Input: part model. Units: mm. Frame: model coordinates. Coordinates: 2 decimals unless noted, no trailing zeros. Loops run counter-clockwise (first coordinate to the right, second up) from the corner with the lowest first, then second, coordinate; pieces in that order, holes last. Notation, with made-up numbers: (47, 70.25) - (100, 70.25) arc R16 ccw to (100, 86.25) - close; hole circle Ø2 at (-33, 50.5). An arc over 180 degrees is marked (long way). Write item = value, one per line. Start each with the question number.
Autodesk Inventor part; units mm, degrees
ref_plane "YZ Plane" through (0, 0, 0) normal (1, 0, 0) x (0, 1, 0)
ref_plane "XZ Plane" through (0, 0, 0) normal (0, 1, 0) x (-1, 0, 0)
ref_plane "XY Plane" through (0, 0, 0) normal (0, 0, 1) x (1, 0, 0)
sketch "Sketch1" plane through (0, 0, 0) normal (0, 0, 1) x (1, 0, 0)
  line L0 (3.175, 0) -> (3.175, 3.175)
  line L1 (3.175, 3.175) -> (-3.175, 3.175)
  line L2 (-3.175, 3.175) -> (-3.175, 0)
  line L3 (5.08, 0) -> (5.08, 5.08)
  line L4 (5.08, 5.08) -> (-5.08, 5.08)
  line L5 (-5.08, 5.08) -> (-5.08, 0)
  line L6 (-5.08, 0) -> (-3.175, 0)
  line L7 (3.175, 0) -> (5.08, 0)
  point P0 (0, 0)
  dimension "d0" = 6.35
  dimension "d1" = 3.175
  dimension "d2" = 10.16
  dimension "d3" = 5.08
extrude "Extrusion1" add sketch "Sketch1" along normal blind 215.9
sketch "Sketch2" plane through (-5.08, 5.08, 0) normal (0, 1, 0) x (1, 0, 0)
  circle A0 centre (5.08, -6.35) radius 1.985
  circle A1 centre (5.08, -209.55) radius 1.985
  circle A2 centre (5.08, -44.45) radius 1.985
  circle A3 centre (5.08, -171.45) radius 1.985
  circle A4 centre (5.08, -95.25) radius 1.985
  circle A5 centre (5.08, -120.65) radius 1.985
  point P0 (5.08, 0)
  dimension "d6" = 3.97
  dimension "d7" = 3.97
  dimension "d8" = 3.97
  dimension "d9" = 3.97
  dimension "d10" = 3.97
  dimension "d11" = 3.97
extrude "Extrusion2" cut sketch "Sketch2" against normal blind 215.9
sketch "Sketch3" plane through (5.08, 0, 0) normal (1, 0, 0) x (0, 0, -1)
  point P0 (0, 0)
sketch "Sketch4" plane through (-5.08, 5.08, 0) normal (0, 1, 0) x (1, 0, 0)
  circle A0 centre (5.08, -6.35) radius 1.985
  circle A1 centre (5.08, -44.45) radius 1.985
  circle A2 centre (5.08, -95.25) radius 1.985
  circle A3 centre (5.08, -120.65) radius 1.985
  circle A4 centre (5.08, -171.45) radius 1.985
  circle A5 centre (5.08, -6.35) radius 5.08
  circle A6 centre (5.08, -44.45) radius 5.08
  line L0 (0, 0) -> (0, -215.9)
  circle A7 centre (5.08, -95.25) radius 5.08
  circle A8 centre (5.08, -120.65) radius 5.08
  circle A9 centre (5.08, -171.45) radius 5.08
  circle A10 centre (5.08, -209.55) radius 1.985
  circle A11 centre (5.08, -209.55) radius 5.08
  point P0 (5.08, 0)
extrude "Extrusion3" add sketch "Sketch4" along normal blind 6.35
properties part number "chassis_brace_jig"
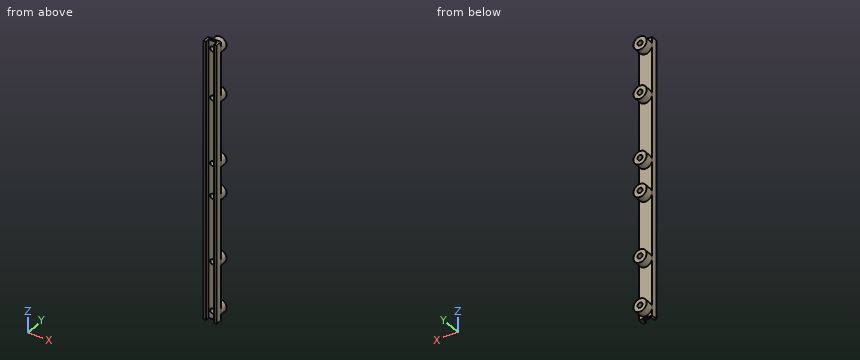
Item 1: Cut plane A-A on y = 9.25. State how many separate pieces and enclosed holes the cut face has, plus the area to 3 significant figures.
Item 2: Pin query (flat end, axial travel): pin 1 (1.5 mm diameter, centred on x = 1.5, z = 56, fed in from -Y) (3 decimals); pin 2 (5 mm diameter, centred on x = -1.5, z = 185, fed in from +Y). Return the tip coordinate at first contact, or that it passes through.
Item 3: Cut plane B-B on z = 27. Return loops of the section in (x, y) (3 decimals).
Item 4: Ray query, line 1 (X direction, y = 1, z = 75.5) (3 decimals); line 2 (X direction, y = 9, z = 95.25) (3 decimals); line 3 (Z direction, x = -2.75, y = 6.5). Return the intervals inside material, ascending.
Recorded:
q1.separate_pieces = 6
q1.enclosed_holes = 6
q1.area = 412 mm²
q2.pin_1 = 3.175
q2.pin_2 = 5.08
q3.outline = (-5.08, 0) - (-3.175, 0) - (-3.175, 3.175) - (3.175, 3.175) - (3.175, 0) - (5.08, 0) - (5.08, 5.08) - (-5.08, 5.08) - close
q4.line_1 = -5.08 to -3.175, 3.175 to 5.08
q4.line_2 = -5.08 to -1.985, 1.985 to 5.08
q4.line_3 = 2.08 to 10.62, 40.18 to 48.72, 90.98 to 99.52, 116.38 to 124.92, 167.18 to 175.72, 205.28 to 213.82
